Can you work these out from the model? Positions are in its coordinate system, mm. Face numbers are marked on the shaded views. A direction names the side the tool comes from. Give positions to 0.01 mm unless a question says otherwise; leave off trailing zeros. Order: outer loops, then holes, each group sorted by start corner. A loop starts at its lowest first (then second) coordinate and runs counter-clockwise, first axis right, second up. Notation, with made-up numbers: (-39.75, 60) - (-10.75, 60) arc R22 ccw to (-10.75, 69) - close; hole circle Ø1 at (-38, 84). An arc over 180 degrees is marked (long way). Answer as CSV lines item,"result".
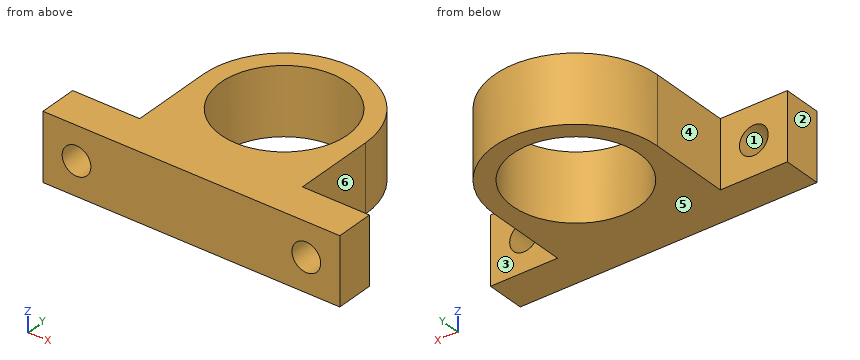
```python
from build123d import *

# Parameters (mm, degrees)
SKETCH_1_R          = 6.6
EXTRUDE_1_DEPTH     = 7
SKETCH_2_R          = 1.5
CUT_EXTRUDE_1_DEPTH = 25.046829313


with BuildPart() as part:
    # 草图1 → 凸台-拉伸1 (new body)
    with BuildSketch(Plane.XY):
        with BuildLine():
            Line((-8.5, 0), (-8.5, -8.5))
            Line((-8.5, -8.5), (-15.5, -8.5))
            Line((-15.5, -8.5), (-15.5, -12.5))
            Line((-15.5, -12.5), (-8.5, -12.5))
            Line((-8.5, -12.5), (8.5, -12.5))
            Line((8.5, -12.5), (15.5, -12.5))
            Line((15.5, -12.5), (15.5, -8.5))
            Line((15.5, -8.5), (8.5, -8.5))
            Line((8.5, -8.5), (8.5, 0))
            ThreePointArc((8.5, 0), (0, 8.5), (-8.5, 0))
        make_face()
        Circle(SKETCH_1_R, mode=Mode.SUBTRACT)
    extrude(amount=EXTRUDE_1_DEPTH)

    # 草图2 → 切除-拉伸1 (cut, through all)
    with BuildSketch(Plane(origin=(0, -8.5, 0), x_dir=(1, 0, 0), z_dir=(0, 1, 0))):
        with Locations(Location((-12, -3.5, 0), (0, 0, 180))):
            Circle(SKETCH_2_R)
        with Locations((12, -3.5)):
            Circle(SKETCH_2_R)
    extrude(amount=-CUT_EXTRUDE_1_DEPTH, mode=Mode.SUBTRACT)


solid = part.part
```
1) I want a section at A-A on z = 3.5. Write out the boundary of the cut face in (x, y).
Answer block:
outline,"(-15.5, -12.5) - (-13.5, -12.5) - (-13.5, -8.5) - (-15.5, -8.5) - close; (-10.5, -12.5) - (10.5, -12.5) - (10.5, -8.5) - (8.5, -8.5) - (8.5, 0) arc R8.5 ccw to (-8.5, 0) - (-8.5, -8.5) - (-10.5, -8.5) - close; (13.5, -12.5) - (15.5, -12.5) - (15.5, -8.5) - (13.5, -8.5) - close; hole circle Ø13.2 at (0, 0)"
2) I want a section at D-D on z = 1.5. Write out the boundary of the cut face in (x, y).
Answer block:
outline,"(-15.5, -12.5) - (15.5, -12.5) - (15.5, -8.5) - (8.5, -8.5) - (8.5, 0) arc R8.5 ccw to (-8.5, 0) - (-8.5, -8.5) - (-15.5, -8.5) - close; hole circle Ø13.2 at (0, 0)"
3) I'm going to push flat-ended pins straight in: P1, Ø3, axis at x = -10.5, z = 5, coming from the +Y side; P2, Ø3.5, axis at y = -4, z = 4, coming from the +X side; P3, Ø10, axis at x = 3.5, y = -0.5, coming from the +Z side; P4, Ø2, axis at y = 3.5, z = 4, coming from the -X side. Where does each tip first touch, or does it pass through?
Answer block:
P1,"y = -8.5"
P2,"x = 8.5"
P3,"z = 7"
P4,"x = -8.12"
4) I need wall thicknesses on line 1 along Y through (x, z) = (0, 3.75); line 2 along X through (y, z) = (-9, 4.25); line 3 along Z through (x, y) = (12, -10.9). Which ranges of each line are inside material? Lowest first, please. Write a range as [from, to].
Answer block:
line 1,"[-12.5, -6.6], [6.6, 8.5]"
line 2,"[-15.5, -13.3], [-10.7, 10.7], [13.3, 15.5]"
line 3,"[0, 2], [5, 7]"
5) I want a section at C-C on y = -5.75. Write out the boundary of the cut face in (x, z).
Answer block:
outline,"(-8.5, 0) - (-3.24, 0) - (-3.24, 7) - (-8.5, 7) - close; (3.24, 0) - (8.5, 0) - (8.5, 7) - (3.24, 7) - close"
6) I want a section at B-B on x = -12. Write out the boundary of the cut face in (y, z).
Answer block:
outline,"(-12.5, 0) - (-8.5, 0) - (-8.5, 2) - (-12.5, 2) - close; (-12.5, 5) - (-8.5, 5) - (-8.5, 7) - (-12.5, 7) - close"
7) Which directions (+Z, -Z, +X, -X, +Y, -Y) give clear straight access to the entire face, cutting with the end or side of a thin tool? Please do the marked faces 4, 5 and 6.
Answer block:
face 4,"+Z, -Z, -X, +Y"
face 5,"-Z, +X, -X, +Y, -Y"
face 6,"+Z, -Z, +X, +Y"
8) If we mould it in two halves opening along X, with no side actions, what happens to the marked faces 1, 2 and 3? For each: +X half, -X half, draft (parallel to the pull), parting line (faces both ways), or undercut.
Answer block:
face 1,"undercut"
face 2,"-X half"
face 3,"draft"
